Here's how the part is built. I have some questions about the finished solid (model axes, mm). A direction names the side the tool comes from. Give positions to 0.01 mm unless a question says otherwise; leave off trailing zeros. Write each loop counter-clockwise with the first axis right and the second up, starting at its lowest first coordinate (ties: lowest second). Pieces come first, ordered by that corner, then holes. Notation, with made-up numbers: (69, -27.5) -> (89, -27.5) arc R18 cw to (89, -21.5) -> close; hole circle Ø2 at (-25, 23). An arc over 180 degrees is marked (long way). Use one line per item in the form item = value.
```python
from build123d import *

# Parameters (mm, degrees)
F0_R      = 63.5
F1_DEPTH  = 25.4
F2_R      = 12.7
F3_DEPTH  = 127
F4_R      = 89.163548
F4_R_2    = 12.7
F5_DEPTH  = 2.54
F5_FACE_R = 89.163548
F7_R      = 38.1


with BuildPart() as f1:
    # F0 (on Top) → F1 (new body)
    with BuildSketch(Plane.XY):
        Circle(F0_R)
    extrude(amount=F1_DEPTH)

    # F2 (on face) → F3 (join)
    with BuildSketch(Plane.XY.offset(25.4)):
        Circle(F2_R)
    extrude(amount=F3_DEPTH)

    # F4 (on face) → F5 (join)
    with BuildSketch(Plane.XY.offset(152.4)):
        Circle(F4_R)
        Circle(F4_R_2, mode=Mode.SUBTRACT)
        Circle(F4_R_2)
    extrude(amount=F5_DEPTH)

    # F5_face (on face) → F8 section 0
    with BuildSketch(Plane.XY.offset(154.94)):
        Circle(F5_FACE_R)
    # F7 (on offset) → F8 section 1
    with BuildSketch(Plane.XY.offset(256.54)):
        Circle(F7_R)
    loft()


solid = f1.part
```
Q1. If I drill on line 1 along Z through (x, y) = (-19.5, -10); line 2 along Z through (x, y) = (-2.5, 59); line 3 along Y through (x, z) = (6, 192.5), over which ranges is the centre line in solid material (lowest first)? Write a range as from..to.
Result set:
line_1 = 0..25.4, 152.4..256.54
line_2 = 0..25.4, 152.4..214.85
line_3 = -70.03..70.03
Q2. Which directions (+Z, -Z, +X, -X, +Y, -Y) give clear straight access to the entire face, cutting with the end or side of a thin tool? Please do faces 1 (the face through (-2.75, -12.4, 88.01)), 2 (the face through (-13.77, -61.99, 12.52)), 3 (the face through (-11.26, -50.69, 229.03)).
Result set:
face_1 = none
face_2 = -Z
face_3 = +Z
Q3. Will these pins go through, and if not, where does the flat tip stop? pin 1 Ø1 at (x, y) = (-16.5, 9.5) entering from -Z; pin 2 Ø2 at (y, z) = (2.5, 184.5) entering from -X; pin 3 Ø1.5 at (x, z) = (8.5, 40.5) entering from -Y; pin 4 Ø1.5 at (x, z) = (-4.5, 170) entering from +Y.
Result set:
pin_1 = 0
pin_2 = -74.77
pin_3 = -10.06
pin_4 = 81.85
Q4. I want a section at C-C, the plane z = 160. Write out the boundary of the cut face in (x, y).
Result set:
outline = circle Ø173.24 at (0, 0)
Q5. I want a section at B-B, the plane z = 111.5. Write out the boundary of the cut face in (x, y), and give its area (3 significant figures).
Result set:
outline = circle Ø25.4 at (0, 0)
area = 507 mm2
Q6. I want a section at A-A, the plane x = 0. Write out the boundary of the cut face in (y, z).
Result set:
outline = (-89.16, 152.4) -> (-12.7, 152.4) -> (-12.7, 25.4) -> (-63.5, 25.4) -> (-63.5, 0) -> (63.5, 0) -> (63.5, 25.4) -> (12.7, 25.4) -> (12.7, 152.4) -> (89.16, 152.4) -> (89.16, 154.94) -> (38.1, 256.54) -> (-38.1, 256.54) -> (-89.16, 154.94) -> close
